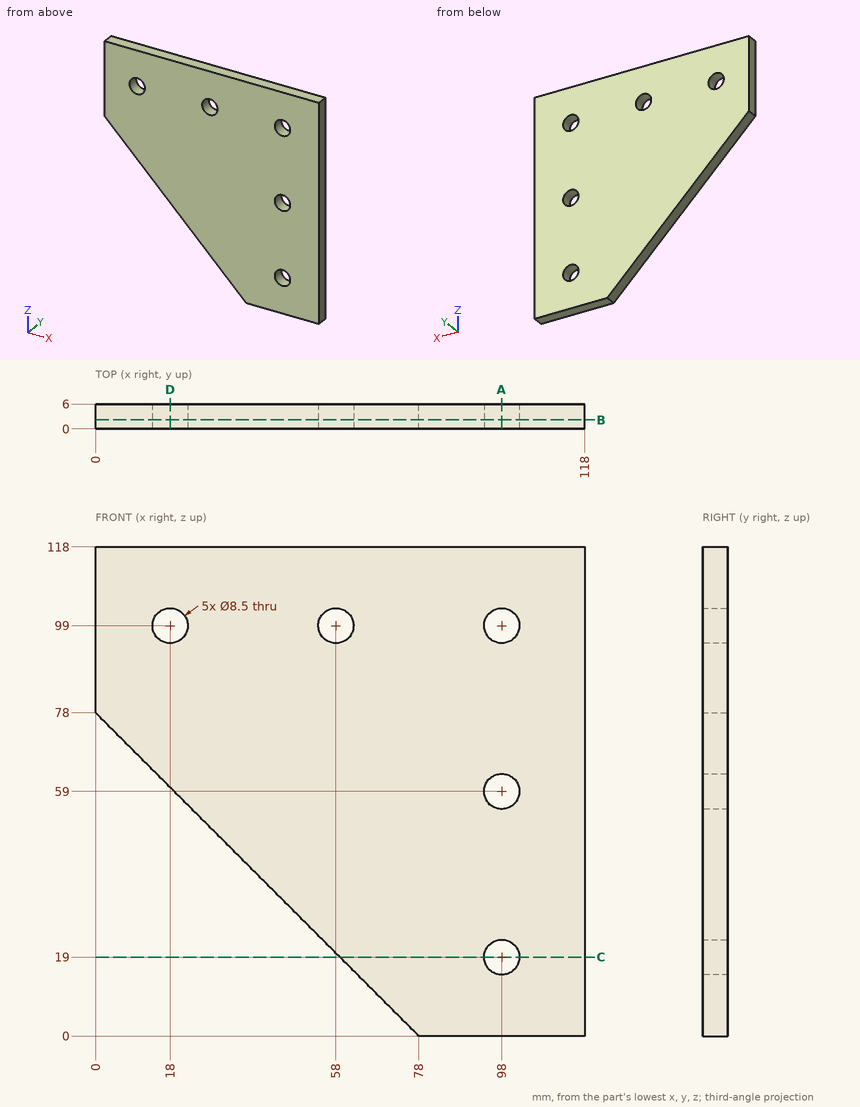
Geometry check sheet. Reference: drawing and pictorial views, mm from the part's lowest x, y, z. Coordinates: 2 decimals unless noted, no trailing zeros. Order: outer loops, then holes, each group sorted by start corner. A loop starts at its lowest first (then second) coordinate and runs counter-clockwise, first axis right, second up. Notation, with made-up numbers: (76, 1) -> (95, 1) arc R32 ccw to (95, 32) -> close; hole circle Ø9 at (-23, -24.75). An arc over 180 degrees is marked (long way). Put each result on its own line as item: value. Start each with the question number.
1) Cross-section at A-A (x = 98). Enter the section's corners in (y, z), plus the area to 3 significant figures.
2) Go/stop test with flat-tipped pins: pin 1 (3 mm diameter, centred on x = 20, y = 0.5, fed in from -Z); pin 2 (2 mm diameter, centred on y = 5, z = 52, fed in from -X). Record where each tip stops, or that it passes through.
3) Material ranges on L1, parallel to X at y = 1.9, z = 99; L2, parallel to X at y = 2.7, z = 100.5; L3, parallel to X at y = 1.7, z = 19, recorded low to high.
4) Cross-section at D-D (x = 18). Enter the section's corners in (y, z), plus the area to 3 significant figures.
5) Cross-section at C-C (z = 19). Enter the section's corners in (x, y), plus the area to 3 significant figures.
6) Cross-section at B-B (y = 2.15). Enter the section's corners in (x, z).
Geometry check:
1. outline: (0, 0) -> (6, 0) -> (6, 14.75) -> (0, 14.75) -> close; (0, 23.25) -> (6, 23.25) -> (6, 54.75) -> (0, 54.75) -> close; (0, 63.25) -> (6, 63.25) -> (6, 94.75) -> (0, 94.75) -> close; (0, 103.25) -> (6, 103.25) -> (6, 118) -> (0, 118) -> close
1. area: 555 mm^2
2. pin 1: stops at z = 56.5
2. pin 2: stops at x = 25
3. L1: x = 0 to 13.75, 22.25 to 53.75, 62.25 to 93.75, 102.25 to 118
3. L2: x = 0 to 14.02, 21.98 to 54.02, 61.98 to 94.02, 101.98 to 118
3. L3: x = 59 to 93.75, 102.25 to 118
4. outline: (0, 60) -> (6, 60) -> (6, 94.75) -> (0, 94.75) -> close; (0, 103.25) -> (6, 103.25) -> (6, 118) -> (0, 118) -> close
4. area: 297 mm^2
5. outline: (59, 0) -> (93.75, 0) -> (93.75, 6) -> (59, 6) -> close; (102.25, 0) -> (118, 0) -> (118, 6) -> (102.25, 6) -> close
5. area: 303 mm^2
6. outline: (0, 78) -> (78, 0) -> (118, 0) -> (118, 118) -> (0, 118) -> close; hole circle Ø8.5 at (18, 99); hole circle Ø8.5 at (58, 99); hole circle Ø8.5 at (98, 19); hole circle Ø8.5 at (98, 59); hole circle Ø8.5 at (98, 99)
